Input: dimensioned drawing with shaded views. Units: mm. Origin: part minimum x, y, z. A direction names the side the tool comes from. Give positions to 0.01 mm unless a question says otherwise; leave off trailing zeros. Order: outer loops, then holes, each group sorted by start corner. A loop starts at its lowest first (then second) coordinate and runs counter-clockwise, first axis right, second up.
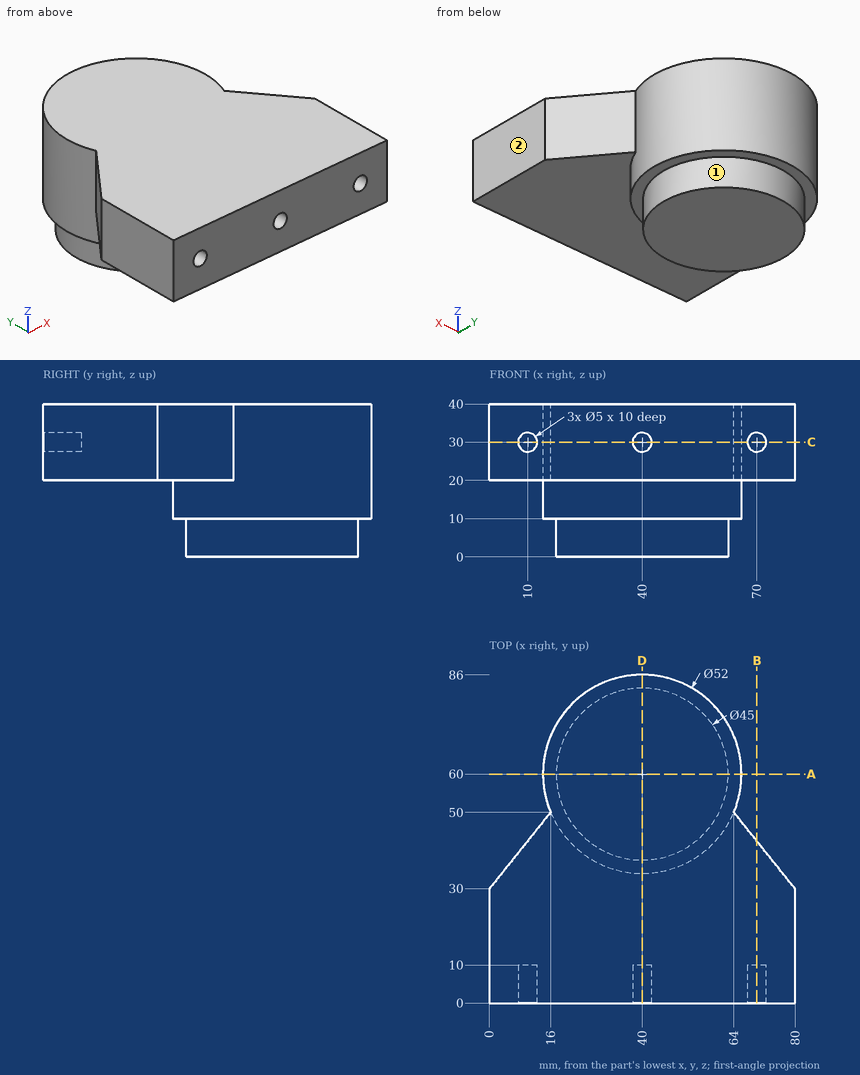
1) Section query B-B, the plane x = 70. Return the cut outline in (y, z), and give its area (3 significant figures).
Report:
outline: (0, 20) - (42.5, 20) - (42.5, 40) - (0, 40) - (0, 32.5) - (10, 32.5) - (10, 27.5) - (0, 27.5) - close
area: 800 mm2
2) Section query A-A, the plane y = 60. Return the cut outline in (x, z).
Report:
outline: (14, 10) - (17.5, 10) - (17.5, 0) - (62.5, 0) - (62.5, 10) - (66, 10) - (66, 40) - (14, 40) - close
3) Section query D-D, the plane x = 40. Return the cut outline in (y, z).
Report:
outline: (0, 20) - (34, 20) - (34, 10) - (37.5, 10) - (37.5, 0) - (82.5, 0) - (82.5, 10) - (86, 10) - (86, 40) - (0, 40) - (0, 32.5) - (10, 32.5) - (10, 27.5) - (0, 27.5) - close
4) Section query C-C, the plane z = 30. Return the cut outline in (x, y).
Report:
outline: (0, 0) - (7.5, 0) - (7.5, 10) - (12.5, 10) - (12.5, 0) - (37.5, 0) - (37.5, 10) - (42.5, 10) - (42.5, 0) - (67.5, 0) - (67.5, 10) - (72.5, 10) - (72.5, 0) - (80, 0) - (80, 30) - (64, 50) arc R26 ccw (long way) to (16, 50) - (0, 30) - close
5) Pin query (flat end, axial travel): pin 1 (6 mm diameter, centred on y = 71, z = 15.5, fed in from +X); pin 2 (10 mm diameter, centred on x = 50.5, z = 22.5, fed in from +Y); pin 3 (5.5 mm diameter, centred on x = 40, z = 29.5, fed in from -Y); pin 4 (1.5 mm diameter, centred on x = 69, z = 29, fed in from -Y). Return the tip coordinate at first contact, or that it passes through.
Report:
pin 1: stops at x = 64.74
pin 2: stops at y = 85.41
pin 3: stops at y = 0
pin 4: stops at y = 10
6) Reachability of the marked faces 1 and 2 from +Z, -Z, +X, -X, +Y, -Y: full face, straight path, thin tool, end or side. Return the list, or none.
Report:
face 1: -Z
face 2: +Z, -Z, +X, +Y, -Y
7) Material intervals for L1, parallel to Z at x = 70, y = 7; L2, parallel to Z at x = 4.5, y = 30.5; L3, parallel to X at y = 70, z = 30.5, sorted ascending.
Report:
L1: z = 20 to 27.5, 32.5 to 40
L2: z = 20 to 40
L3: x = 16 to 64
